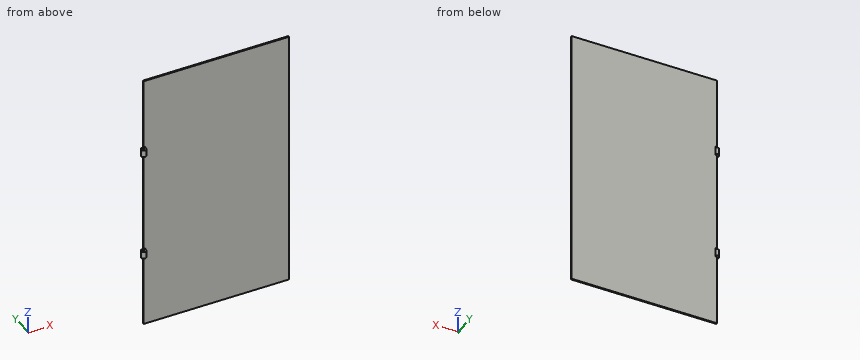
```python
from build123d import *

# Parameters (mm, degrees)
SKETCH1_W               = 300
SKETCH1_H               = 550
BOSS_EXTRUDE1_DEPTH     = 2.5
SKETCH3_R               = 5
SKETCH3_R_2             = 1.245895
BOSS_EXTRUDE2_DEPTH     = 15
SKETCH4_R               = 5
CUT_EXTRUDE1_DEPTH      = 2.5
MIRROR3_COPY_1_SKETCH_R = 5
MIRROR3_COPY_1_DEPTH    = 2.5


with BuildPart() as part:
    # Sketch1 → Boss-Extrude1 (new body)
    with BuildSketch(Plane(origin=(0, 0, 0), x_dir=(1, 0, 0), z_dir=(0, 1, 0))):
        with Locations((150, 275)):
            Rectangle(SKETCH1_W, SKETCH1_H)
    extrude(amount=BOSS_EXTRUDE1_DEPTH)

    # Sketch3 → Boss-Extrude2 (add)
    with BuildSketch(Plane.XY.offset(-152.5)):
        with Locations((-0.485034728, -1.147604315)):
            Circle(SKETCH3_R)
        with Locations(Location((-0.485034728, -1.147604315, 0), (0, 0, 67.08866))):
            Circle(SKETCH3_R_2, mode=Mode.SUBTRACT)
    boss_extrude2 = extrude(amount=-BOSS_EXTRUDE2_DEPTH)

    # Mirror1: Boss-Extrude2 across plane
    add(boss_extrude2.mirror(Plane.XY.offset(-275)))

    # Sketch4 → Cut-Extrude1 (cut)
    with BuildSketch(Plane.XY.offset(-152.5)):
        with Locations((-0.485034728, -1.147604315)):
            Circle(SKETCH4_R)
    cut_extrude1 = extrude(amount=CUT_EXTRUDE1_DEPTH, mode=Mode.SUBTRACT)

    # Mirror2: Cut-Extrude1 across plane
    add(cut_extrude1.mirror(Plane.XY.offset(-160)), mode=Mode.SUBTRACT)

    # Mirror3: Cut-Extrude1 across plane
    add(cut_extrude1.mirror(Plane.XY.offset(-275)), mode=Mode.SUBTRACT)

    # Mirror3 copy 1 sketch → Mirror3 copy 1 (cut)
    with BuildSketch(Plane.XY.offset(-382.5)):
        with Locations((-0.485034728, -1.147604315)):
            Circle(MIRROR3_COPY_1_SKETCH_R)
    extrude(amount=MIRROR3_COPY_1_DEPTH, mode=Mode.SUBTRACT)


solid = part.part
```
Source: CAD feature listing. Evaluate the final solid. Frame: model axes, mm. Give positions to 0.01 mm unless a question says otherwise; leave off trailing zeros. Write each loop counter-clockwise with the first axis right and the second up, starting at its lowest first coordinate (ties: lowest second). Pieces come first, ordered by that corner, then holes.
1. Section query B-B (x = 59.5). Return the cut outline in (y, z), then the cut area to 4 significant figures.
2. Section query A-A (z = -427). Return the cut outline in (x, y), then the cut area to 3 significant figures.
3. First-contact query: pin 1 (1.2 mm diameter, centred on y = 1, z = -286, fed in from -X); pin 2 (3 mm diameter, centred on x = 126.5, z = -344, fed in from -Y); pin 3 (1.5 mm diameter, centred on x = 185, z = -94, fed in from +Y). Flat tips, straight axial feed; report the tip coordinate or a pass-through.
4. Material intervals for line 1 along X through (y, z) = (1.5, -526.5); line 2 along Y through (x, z) = (9.5, -366), sorted ascending.
Output values:
1. outline: (0, -550) - (2.5, -550) - (2.5, 0) - (0, 0) - close
1. area: 1,375 mm2
2. outline: (0, 0) - (300, 0) - (300, 2.5) - (0, 2.5) - close
2. area: 750 mm2
3. pin 1: stops at x = 0
3. pin 2: stops at y = 0
3. pin 3: stops at y = 2.5
4. line 1: x = 0 to 300
4. line 2: y = 0 to 2.5
